Read the model definition and answer for the solid it produces. Units are mm, in the model's axes. A direction names the side the tool comes from. Round coordinates to 2 decimals unless told otherwise and drop trailing zeros. Write each loop counter-clockwise with the first axis right and the second up, starting at its lowest first coordinate (ties: lowest second). Pieces come first, ordered by that corner, then holes.
from build123d import *

# Parameters (mm, degrees)
SKETCH1_W                = 4.983520766
SKETCH1_H                = 2.5
SKETCH1_R                = 0.3
BOSS_EXTRUDE1_DEPTH      = 1
SKETCH4_R                = 0.5
SKETCH4_W                = 1
SKETCH4_H                = 2.5
BOSS_EXTRUDE2_DEPTH      = 1
SKETCH4_3_R              = 0.5
BOSS_EXTRUDE3_DEPTH      = 1.5
BOSS_EXTRUDE4_DEPTH      = 1
BOSS_EXTRUDE4_DEPTH_BACK = 1
BOSS_EXTRUDE5_DEPTH      = 1.5
BOSS_EXTRUDE5_DEPTH_BACK = 1.5
SKETCH5_4_W              = 4.983520766
SKETCH5_4_H              = 1.5
SKETCH7_R                = 0.5
BOSS_EXTRUDE6_DEPTH      = 1.5


with BuildPart() as part:
    # Sketch1 → Boss-Extrude1 (new body)
    with BuildSketch(Plane.XY):
        with Locations((1.3, 0)):
            Rectangle(SKETCH1_W, SKETCH1_H)
        Circle(SKETCH1_R, mode=Mode.SUBTRACT)
        with Locations((1.3, 0)):
            Circle(SKETCH1_R, mode=Mode.SUBTRACT)
        with Locations((2.6, 0)):
            Circle(SKETCH1_R, mode=Mode.SUBTRACT)
    extrude(amount=-BOSS_EXTRUDE1_DEPTH)

    # Sketch4 → Boss-Extrude2 (add)
    # profile 1 of 4: a face of its own
    with BuildSketch(Plane.ZY.offset(1.191760383)):
        Polygon((0, 1.25), (0, 7.6), (-8.75, 7.6), (-8.75, -7.6), (0, -7.6), (0, -1.25), (-1, -1.25), (-1, 1.25), align=None)
        with Locations((-7.2, -6)):
            Circle(SKETCH4_R, mode=Mode.SUBTRACT)
        with Locations((-7.2, 6)):
            Circle(SKETCH4_R, mode=Mode.SUBTRACT)
    # profile 2 of 4: a face of its own
    with BuildSketch(Plane.ZY.offset(1.191760383)):
        with Locations((-7.2, 6)):
            Circle(SKETCH4_R)
    # profile 3 of 4: a face of its own
    with BuildSketch(Plane.ZY.offset(1.191760383)):
        with Locations((-7.2, -6)):
            Circle(SKETCH4_R)
    # profile 4 of 4: a face of its own
    with BuildSketch(Plane.ZY.offset(1.191760383)):
        with Locations((-0.5, 0)):
            Rectangle(SKETCH4_W, SKETCH4_H)
    extrude(amount=BOSS_EXTRUDE2_DEPTH)

    # Sketch4_3 → Boss-Extrude3 (add)
    with BuildSketch(Plane.ZY.offset(1.191760383)):
        with Locations((-7.2, -6)):
            Circle(SKETCH4_3_R)
        with Locations((-7.2, 6)):
            Circle(SKETCH4_3_R)
    extrude(amount=BOSS_EXTRUDE3_DEPTH)


with BuildPart() as body_2:
    # Mirror3: mirrored copy
    add(part.part.mirror(Plane.XY.offset(0.5)))


with BuildPart() as part_1:
    add(part.part)

    add(body_2.part)  # Boss-Extrude4 merges body 2
    # Sketch5 → Boss-Extrude4 (add, two sides: drawn at the far end of the back side and taken through both)
    with BuildSketch(Plane.XY.offset(0.5).offset(-BOSS_EXTRUDE4_DEPTH_BACK)):
        Polygon((-2.191760383, -7.6), (-1.191760383, -7.6), (-1.191760383, -1.25), (-1.191760383, 1.25), (-1.191760383, 7.6), (-2.191760383, 7.6), align=None)
    extrude(amount=BOSS_EXTRUDE4_DEPTH + BOSS_EXTRUDE4_DEPTH_BACK)

    # Sketch5_4 → Boss-Extrude5 (add, two sides: drawn at the far end of the back side and taken through both)
    with BuildSketch(Plane.XY.offset(0.5).offset(-BOSS_EXTRUDE5_DEPTH_BACK)):
        with Locations((1.3, -2)):
            Rectangle(SKETCH5_4_W, SKETCH5_4_H)
        with Locations((1.3, 2)):
            Rectangle(SKETCH5_4_W, SKETCH5_4_H)
    extrude(amount=BOSS_EXTRUDE5_DEPTH + BOSS_EXTRUDE5_DEPTH_BACK)

    # Sketch7 → Boss-Extrude6 (add)
    # profile 1 of 2: a face of its own
    with BuildSketch(Plane.ZY.offset(2.191760383)):
        with BuildLine():
            Line((-8.75, -7.5), (-7.2, -7.5))
            Line((-7.2, -7.5), (9.75, -7.6))
            Line((9.75, -7.6), (9.75, -6.05))
            Line((9.75, -6.05), (8.698032426, -6.044313689))
            ThreePointArc((8.698032426, -6.044313689), (8.197297337, -6.499992696), (7.701517624, -6.038927122))
            Line((7.701517624, -6.038927122), (0.5, -6))
            Line((0.5, -6), (0.5, -4.5))
            Line((0.5, -4.5), (-8.75, -4.5))
            Line((-8.75, -4.5), (-8.75, -7.5))
        make_face()
        with Locations((-7.2, -6)):
            Circle(SKETCH7_R, mode=Mode.SUBTRACT)
    # profile 2 of 2: a face of its own
    with BuildSketch(Plane.ZY.offset(2.191760383)):
        with BuildLine():
            Line((-8.75, 7.5), (-8.75, 4.5))
            Line((-8.75, 4.5), (0.5, 4.5))
            Line((0.5, 4.5), (0.5, 6))
            Line((0.5, 6), (7.7, 6))
            ThreePointArc((7.7, 6), (8.2, 6.5), (8.7, 6))
            Line((8.7, 6), (9.75, 6))
            Line((9.75, 6), (9.75, 7.5))
            Line((9.75, 7.5), (-8.75, 7.5))
        make_face()
        with Locations((-7.2, 6)):
            Circle(SKETCH7_R, mode=Mode.SUBTRACT)
    extrude(amount=BOSS_EXTRUDE6_DEPTH)


solid = part_1.part
Q1. Section A-A (x = 0) is taken. Determine the outline of the cut face in (y, z), then the cut area to 3 significant figures.
Verdict:
outline: (-2.75, -1) - (-0.3, -1) - (-0.3, 0) - (-1.25, 0) - (-1.25, 1) - (-0.3, 1) - (-0.3, 2) - (-2.75, 2) - close; (0.3, -1) - (2.75, -1) - (2.75, 2) - (0.3, 2) - (0.3, 1) - (1.25, 1) - (1.25, 0) - (0.3, 0) - close
area: 12.8 mm2
Q2. Flat-ended cylindrical pins translate along their axes: pin 1 Ø0.8 at (y, z) = (0, 0.5) entering from +X; pin 2 Ø0.8 at (x, z) = (-3, 2.5) entering from -Y; pin 3 Ø0.9 at (x, z) = (1, 0.5) entering from -Y. Find the tip coordinate at first contact, or state that the pin passes through.
Verdict:
pin 1: stops at x = -1.19
pin 2: stops at y = -7.56
pin 3: stops at y = -2.75
Q3. Section B-B (y = 2) is taken. Determine the outline of the cut face in (x, z), then the cut area to 3 significant figures.
Verdict:
outline: (-2.19, -8.75) - (-1.19, -8.75) - (-1.19, -1) - (3.79, -1) - (3.79, 2) - (-1.19, 2) - (-1.19, 9.75) - (-2.19, 9.75) - close
area: 33.5 mm2
Q4. Determine the mould class of faces 6 (the cylindrical face through (-3.185, 5.808, -6.738)), 7 (the flat face through (-2, 7.6, 1)), 8 (the flat face through (2, 0, -1)) for opening direction Z: pulls with the +Z half, pulls with the -Z half, needs draft (parallel to the pull), parting line crosses it, or undercut.
Verdict:
face 6: undercut
face 7: needs draft
face 8: pulls with the -Z half
Q5. Section D-D (y = 0) is taken. State how many separate pieces and enclosed holes the cut face has, then the cut area to 3 significant figures.
Verdict:
separate pieces: 7
enclosed holes: 0
area: 24.9 mm2
Q6. Straight lines are drawn through the part: probe 1 along Z at (x, y) = (1, -0.5); probe 2 along Y at (x, z) = (2.6, -0.55); probe 3 along X at (y, z) = (-3.25, -7). For each, find the intervals that lie inside material, in ascending order.
Verdict:
probe 1: z = -1 to 0, 1 to 2
probe 2: y = -2.75 to -0.3, 0.3 to 2.75
probe 3: x = -2.19 to -1.19
Q7. Which of the six approach directions +Z, -Z, +X, -X, +Y, -Y give full straight-line access (tool end or side, diameter ignored) to faces 1 (the flat face through (-3.692, 6, -2)), 2 (the cylindrical face through (-3.185, -5.85, -6.723)), 3 (the flat face through (1, -2.75, 0)), 4 (the flat face through (-3, -4.5, -4)), 5 (the flat face through (2, 0, 0))?
Verdict:
face 1: +Z, -Z, -X, +Y, -Y
face 2: -X
face 3: +Z, -Z, +X, -Y
face 4: +Z, -Z, -X
face 5: +X
